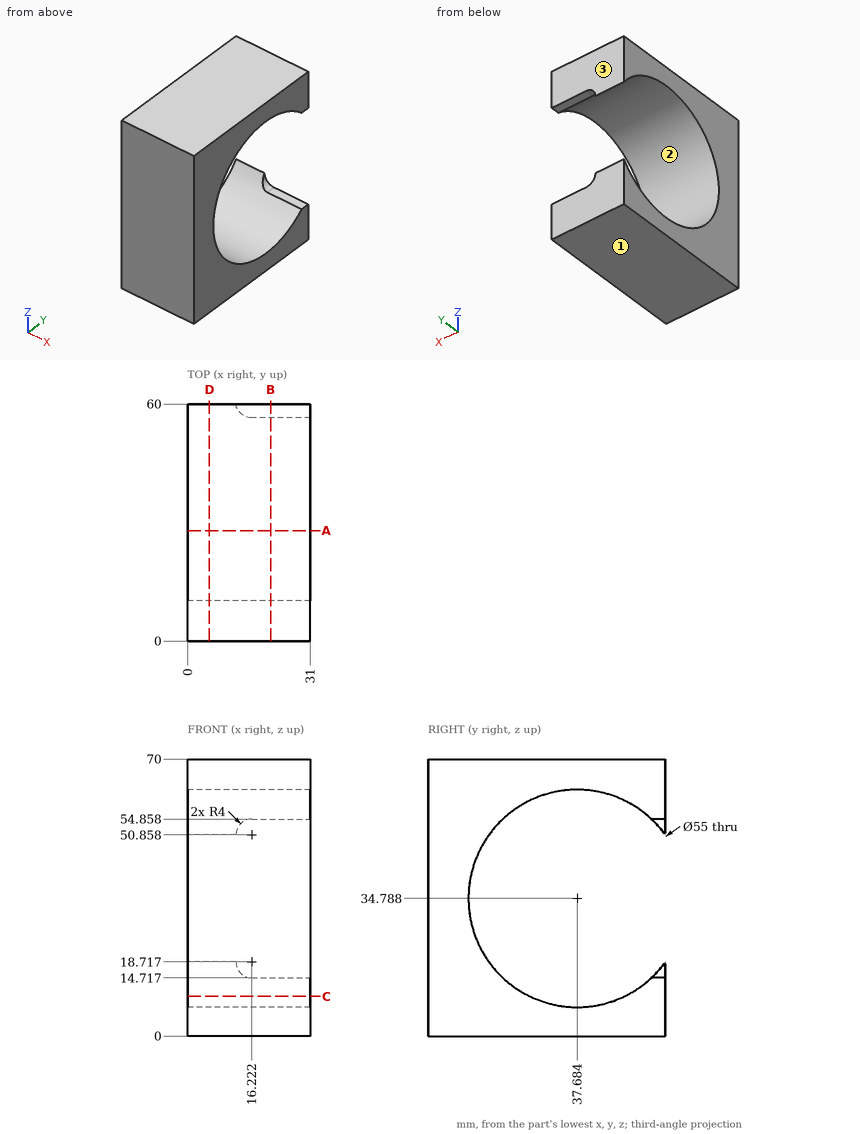
Design review of the part shown in the three views and the two pictorial views. Dimensions are in mm from the part's minimum x, y and z. Coordinates: 2 decimals unless noted, no trailing zeros. Order: outer loops, then holes, each group sorted by start corner. A loop starts at its lowest first (then second) coordinate and runs counter-clockwise, first axis right, second up.
Item 1: For line 1 (Z direction, x = 8.5, y = 37); line 2 (Z direction, x = 12, y = 12.5) (1 decimal); line 3 (Y direction, x = 4.5, z = 54), list the stretches that pass through material, from the lowest coordinate up.
Item 2: Take a section at A-A, the plane y = 28. Write out the cut boundary in (x, z), then the cut area to 3 significant figures.
Item 3: The part is to be moulded in two halves that separate along Z. For the marked faces 1, 2 and 3, say which applies: pulls with the +Z half, pulls with the -Z half, needs draft (parallel to the pull), parting line crosses it, or undercut.
Item 4: For pin 1 Ø1.5 at (x, z) = (12.5, 37.5) entering from -Y; pin 2 Ø5 at (x, z) = (4.5, 36) entering from +Y, all flat-tipped, find the tip position at first contact; note any pin that passes through.
Item 5: Take a section at B-B, the plane x = 21. Write out the cut boundary in (y, z) (1 decimal).
Item 6: Take a section at D-D, the plane x = 5.5. Write out the cut boundary in (y, z) (1 decimal).
Item 7: Take a section at C-C, the plane z = 10. Write out the cut boundary in (x, y).
The answers:
1. line 1: z = 0 to 7.3, 62.28 to 70
1. line 2: z = 0 to 23.7, 45.8 to 70
1. line 3: y = 0 to 18.01, 57.36 to 60
2. outline: (0, 0) - (31, 0) - (31, 9.05) - (0, 9.05) - close; (0, 60.53) - (31, 60.53) - (31, 70) - (0, 70) - close
2. area: 574 mm2
3. face 1: pulls with the -Z half
3. face 2: undercut
3. face 3: needs draft
4. pin 1: stops at y = 0
4. pin 2: stops at y = 10.44
5. outline: (0, 0) - (60, 0) - (60, 14.7) - (56.5, 14.7) arc R27.5 cw (long way) to (56.5, 54.9) - (60, 54.9) - (60, 70) - (0, 70) - close
6. outline: (0, 0) - (60, 0) - (60, 18.7) arc R27.5 cw (long way) to (60, 50.9) - (60, 70) - (0, 70) - close
7. outline: (0, 0) - (31, 0) - (31, 25.78) - (0, 25.78) - close; (0, 49.59) - (31, 49.59) - (31, 60) - (0, 60) - close
